Job drawing, mm, ordinate dimensions from the low corner. One solid piece. A direction names the side the tool comes from. Give positions to 0.01 mm unless a question says otherwise; leave off trailing zeros. Order: outer loops, then holes, each group sorted by start corner. A loop starts at its lowest first (then second) coordinate and runs counter-clockwise, first axis right, second up. Notation, with made-up numbers: (-1, 69.25) - (58, 69.25) arc R22 cw to (58, 77.25) - close; hole circle Ø4 at (-12.5, 33). An arc over 180 degrees is marked (long way). Use one line per item in the form item = value. Start each with the question number.
1. Tool access for the marked faces 4, 5 and 6: list every direction of +Z, -Z, +X, -X, +Y, -Y with a clear straight run to the whole face (end or side of a thin tool).
2. Band-saw the part on D-D, the plane x = 11. List the corners of the cut face in (y, z).
3. Drill centre lines: line 1 (Y direction, x = 1.25, z = 8.5); line 2 (Z direction, x = 10, y = 5.5); line 3 (Y direction, x = 3.5, z = 6.25). Where is each one in solid material? Low to high.
4. Pull direction Z, two halves, no side cores. Call the marked faces 1, 2 and 3: +Z half, -Z half, draft (parallel to the pull), parting line (faces both ways), or undercut.
5. Band-saw the part on A-A, the plane x = 8. List the corners of the cut face in (y, z), plus the area to 3 significant figures.
6. Band-saw the part on C-C, the plane y = 8.5. List the corners of the cut face in (x, z).
7. Band-saw the part on B-B, the plane z = 8. List the corners of the cut face in (x, y).
8. Pin check, flat tips, straight feed: P1, Ø1.2, axis at x = 7.5, z = 7, coming from the -Y side; P2, Ø4.5, axis at x = 9, y = 1, coming from the -Z side; P3, Ø2, axis at y = 9.5, z = 6, coming from the +X side; P4, Ø3, axis at y = 18.5, z = 14, coming from the +X side. Stop position of each tip, or through.
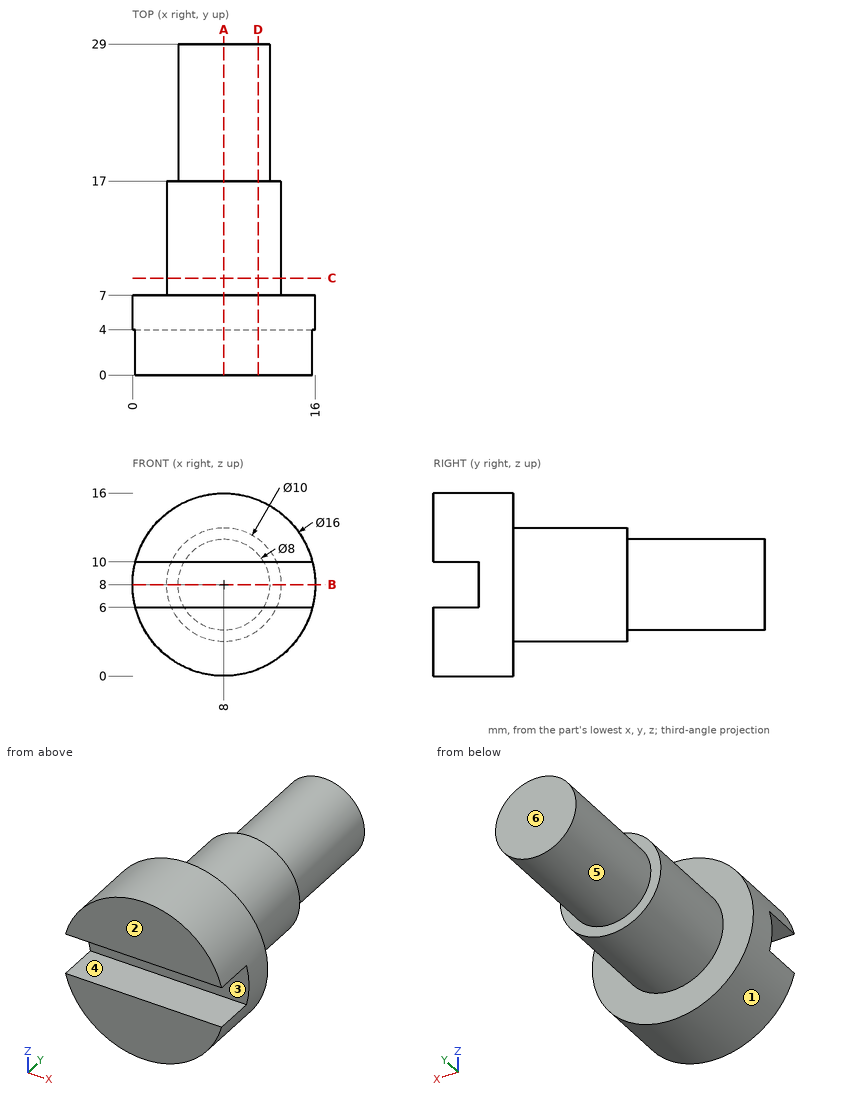
From the geometry:
q1.face_4 = +X, -X, -Y
q1.face_5 = +Y
q1.face_6 = +Z, -Z, +X, -X, +Y
q2.outline = (0, 0.58) - (7, 0.58) - (7, 4) - (17, 4) - (17, 5.35) - (29, 5.35) - (29, 10.65) - (17, 10.65) - (17, 12) - (7, 12) - (7, 15.42) - (0, 15.42) - (0, 10) - (4, 10) - (4, 6) - (0, 6) - close
q3.line_1 = 4 to 7
q3.line_2 = 0.25 to 15.75
q3.line_3 = 4 to 17
q4.face_1 = parting line
q4.face_2 = draft
q4.face_3 = undercut
q5.outline = (0, 0) - (7, 0) - (7, 3) - (17, 3) - (17, 4) - (29, 4) - (29, 12) - (17, 12) - (17, 13) - (7, 13) - (7, 16) - (0, 16) - (0, 10) - (4, 10) - (4, 6) - (0, 6) - close
q5.area = 292 mm²
q6.outline = circle Ø10 at (8, 8)
q7.outline = (0, 4) - (16, 4) - (16, 7) - (13, 7) - (13, 17) - (12, 17) - (12, 29) - (4, 29) - (4, 17) - (3, 17) - (3, 7) - (0, 7) - close
q8.P1 = 4
q8.P2 = 0
q8.P3 = 12.9
q8.P4 = through
